The listing builds one solid part. Answer for the finished solid, in the listing's coordinates (mm). A direction names the side the tool comes from. Round coordinates to 2 decimals unless told otherwise and drop trailing zeros. Write each loop counter-clockwise with the first axis right and the second up, starting at its lowest first coordinate (ties: lowest second). Pieces come first, ordered by that corner, then holes. Notation, with made-up numbers: (42, 56) - (74, 56) arc R25 ccw to (74, 72) - close; hole circle Ø8 at (6.5, -28). An arc over 180 degrees is marked (long way). Use a Markdown table: item, result. Add a question column.
1) A cutting plane is placed at D-D (x = 14.5). Give the vertices of the cut face in (y, z), then the cut area to 3 significant figures.
2) Find the intervals of material crossed by probe 1 along Y at (x, z) = (51, 8.75); probe 2 along X at (y, z) = (51, 4); probe 3 along Y at (x, z) = (51, 6), in increasing order. Write a range as from..to.
3) Determine the mould class of faces 6 (the flat face through (22, 55, 4)), 7 (the flat face through (53, 54.4, 8)), 8 (the cylindrical face through (42.23, 50.94, 4.29)) for opening direction Z: +Z half, -Z half, draft (parallel to the pull), parting line (faces both ways), or undercut.
4) A cutting plane is placed at B-B (z = 4). Give the vertices of the cut face in (x, y).
5) A cutting plane is placed at A-A (y = 45.25). Give the vertices of the cut face in (x, z), then the cut area to 3 significant figures.
6) A tool of negligible diameter and unlimited length cuts with its end or side. For faces 1 (the flat face through (-9, 27.5, 8)), 2 (the flat face through (53, 27.6, 8)), 3 (the flat face through (22, 47, 4)), 4 (the flat face through (21.6, 47.4, 8)), 5 (the flat face through (-8.9, 54.5, 8)), from which of +Z, -Z, +X, -X, +Y, -Y can it reach the whole face along a straight path? Write none if from no direction.
7) A cutting plane is placed at C-C (x = 4). Give the vertices of the cut face in (y, z), then the cut area to 3 significant figures.
8) Each of these flat-tipped pins is pushed along its axis until it touches: P1, Ø4, axis at x = 51, y = 29.5, coming from the +Z side; P2, Ø2, axis at x = -7, y = 29.5, coming from the +Z side; P3, Ø1, axis at x = 18, z = 2, coming from the -Y side; P4, Ø8, axis at x = 43.5, y = 38.5, coming from the +Z side. Where does it stop, or does it pass through?
```python
from build123d import *

# Parameters (mm, degrees)
SCHIZZO1_W                   = 28
SCHIZZO1_H                   = 39
ESTRUSIONE_ESTRUSIONE1_DEPTH = 8
SCHIZZO2_R                   = 1.75
TAGLIO_ESTRUSIONE1_DEPTH     = 20
ESTRUSIONE_ESTRUSIONE2_DEPTH = 8
SCHIZZO4_R                   = 2.5
SCHIZZO4_R_2                 = 1.25
ESTRUSIONE_ESTRUSIONE3_DEPTH = 2
SCHIZZO5_R                   = 1.25
TAGLIO_ESTRUSIONE2_DEPTH     = 78.144345224
SCHIZZO6_W                   = 28
SCHIZZO6_H                   = 8
TAGLIO_ESTRUSIONE3_DEPTH     = 10
SCHIZZO7_W                   = 28
SCHIZZO7_H                   = 8
ESTRUSIONE_ESTRUSIONE4_DEPTH = 8
SCHIZZO8_W                   = 44
SCHIZZO8_H                   = 47
TAGLIO_ESTRUSIONE4_DEPTH     = 8
SCHIZZO9_R                   = 2.25
TAGLIO_ESTRUSIONE5_DEPTH     = 8


with BuildPart() as part:
    # Schizzo1 → Estrusione-Estrusione1 (new body)
    with BuildSketch(Plane.XY):
        Polygon((0, 0), (0, 55), (44, 55), (44, 0), (36, 0), (8, 0), align=None)
        with Locations((22, 27.5)):
            Rectangle(SCHIZZO1_W, SCHIZZO1_H, mode=Mode.SUBTRACT)
    extrude(amount=ESTRUSIONE_ESTRUSIONE1_DEPTH)

    # Schizzo2 → Taglio-Estrusione1 (cut)
    with BuildSketch(Plane.XZ):
        with Locations((4, 4)):
            Circle(SCHIZZO2_R)
        with Locations((40, 4)):
            Circle(SCHIZZO2_R)
    extrude(amount=-TAGLIO_ESTRUSIONE1_DEPTH, mode=Mode.SUBTRACT)

    # Schizzo3 → Estrusione-Estrusione2 (add)
    with BuildSketch(Plane.XY.offset(8)):
        Polygon((-9.5, 55), (53.5, 55), (53.5, 27), (36, 27), (36, 47), (8, 47), (8, 27), (-9.5, 27), align=None)
    extrude(amount=-ESTRUSIONE_ESTRUSIONE2_DEPTH)

    # Schizzo4 → Estrusione-Estrusione3 (add)
    # profile 1 of 4: a face of its own
    with BuildSketch(Plane.XY.offset(8)):
        with Locations(Location((-7, 52.5, 0), (0, 0, 180))):
            Circle(SCHIZZO4_R)
        with Locations((-7, 52.5)):
            Circle(SCHIZZO4_R_2, mode=Mode.SUBTRACT)
    # profile 2 of 4: a face of its own
    with BuildSketch(Plane.XY.offset(8)):
        with Locations(Location((-7, 29.5, 0), (0, 0, 180))):
            Circle(SCHIZZO4_R)
        with Locations((-7, 29.5)):
            Circle(SCHIZZO4_R_2, mode=Mode.SUBTRACT)
    # profile 3 of 4: a face of its own
    with BuildSketch(Plane.XY.offset(8)):
        with Locations((51, 29.5)):
            Circle(SCHIZZO4_R)
        with Locations((51, 29.5)):
            Circle(SCHIZZO4_R_2, mode=Mode.SUBTRACT)
    # profile 4 of 4: a face of its own
    with BuildSketch(Plane.XY.offset(8)):
        with Locations((51, 52.5)):
            Circle(SCHIZZO4_R)
        with Locations((51, 52.5)):
            Circle(SCHIZZO4_R_2, mode=Mode.SUBTRACT)
    extrude(amount=ESTRUSIONE_ESTRUSIONE3_DEPTH)

    # Schizzo5 → Taglio-Estrusione2 (cut, through all)
    with BuildSketch(Plane.XY.offset(8)):
        with Locations((-7, 52.5)):
            Circle(SCHIZZO5_R)
        with Locations((-7, 29.5)):
            Circle(SCHIZZO5_R)
        with Locations((51, 52.5)):
            Circle(SCHIZZO5_R)
        with Locations((51, 29.5)):
            Circle(SCHIZZO5_R)
    extrude(amount=-TAGLIO_ESTRUSIONE2_DEPTH, mode=Mode.SUBTRACT)

    # Schizzo6 → Taglio-Estrusione3 (cut)
    with BuildSketch(Plane.XY.offset(8)):
        with Locations((22, 51)):
            Rectangle(SCHIZZO6_W, SCHIZZO6_H)
    extrude(amount=-TAGLIO_ESTRUSIONE3_DEPTH, mode=Mode.SUBTRACT)

    # Schizzo7 → Estrusione-Estrusione4 (add)
    with BuildSketch(Plane.XY.offset(8)):
        with Locations((22, 51)):
            Rectangle(SCHIZZO7_W, SCHIZZO7_H)
    extrude(amount=-ESTRUSIONE_ESTRUSIONE4_DEPTH)

    # Schizzo8 → Taglio-Estrusione4 (cut)
    with BuildSketch(Plane.XY.offset(8)):
        with Locations((22, 23.5)):
            Rectangle(SCHIZZO8_W, SCHIZZO8_H)
    extrude(amount=-TAGLIO_ESTRUSIONE4_DEPTH, mode=Mode.SUBTRACT)

    # Schizzo9 → Taglio-Estrusione5 (cut)
    with BuildSketch(Plane.XZ.offset(-47)):
        with Locations(Location((4, 4, 0), (0, 0, 270))):
            Circle(SCHIZZO9_R)
        with Locations(Location((40, 4, 0), (0, 0, 270))):
            Circle(SCHIZZO9_R)
    extrude(amount=-TAGLIO_ESTRUSIONE5_DEPTH, mode=Mode.SUBTRACT)


solid = part.part
```
Entries:
| question | item | result |
|---|---|---|
| 1 | outline | (47, 0) - (55, 0) - (55, 8) - (47, 8) - close |
| 1 | area | 64.0 mm² |
| 2 | probe 1 | y = 27..28.25, 30.75..32, 50..51.25, 53.75..55 |
| 2 | probe 2 | x = -9.5..1.75, 6.25..37.75, 42.25..53.5 |
| 2 | probe 3 | y = 27..28.25, 30.75..51.25, 53.75..55 |
| 3 | face 6 | draft |
| 3 | face 7 | +Z half |
| 3 | face 8 | undercut |
| 4 | outline | (-9.5, 27) - (0, 27) - (0, 47) - (1.75, 47) - (1.75, 55) - (-9.5, 55) - close; (6.25, 47) - (37.75, 47) - (37.75, 55) - (6.25, 55) - close; (42.25, 47) - (44, 47) - (44, 27) - (53.5, 27) - (53.5, 55) - (42.25, 55) - close; hole circle Ø2.5 at (-7, 29.5); hole circle Ø2.5 at (-7, 52.5); hole circle Ø2.5 at (51, 29.5); hole circle Ø2.5 at (51, 52.5) |
| 5 | outline | (-9.5, 0) - (0, 0) - (0, 8) - (-9.5, 8) - close; (44, 0) - (53.5, 0) - (53.5, 8) - (44, 8) - close |
| 5 | area | 152 mm² |
| 6 | face 1 | +Z, -X, -Y |
| 6 | face 2 | +Z, +X, -Y |
| 6 | face 3 | +Z, -Z, -Y |
| 6 | face 4 | +Z |
| 6 | face 5 | +Z, -X, +Y |
| 7 | outline | (47, 0) - (55, 0) - (55, 1.75) - (47, 1.75) - close; (47, 6.25) - (55, 6.25) - (55, 8) - (47, 8) - close |
| 7 | area | 28.0 mm² |
| 8 | P1 | stops at z = 10 |
| 8 | P2 | passes through |
| 8 | P3 | stops at y = 47 |
| 8 | P4 | stops at z = 8 |
